Could you check a few things on this model? Use its own coordinates, in mm. Face numbers are marked on the shaded views. A direction names the side the tool comes from. Give positions to 0.01 mm unless a question says otherwise; leave off trailing zeros. Loops run counter-clockwise (first coordinate to the right, second up) from the corner with the lowest first, then second, coordinate; pieces in that order, holes last. Notation, with made-up numbers: (58.5, -25) -> (72.5, -25) arc R14 ccw to (72.5, -4) -> close; hole circle Ø3 at (-3.5, 62.5). An arc over 180 degrees is marked (long way). Write each question's results on one line, items separated by ' | '. Start each with the question number.
Q1. If I drill on line 1 along Z through (x, y) = (84.5, 7.5); line 2 along Y through (x, z) = (11, 51); line 3 along X through (y, z) = (27, 42.5), over which ranges is the centre line in solid material (lowest first)?
Q2. If we section it at B-B, the plane y = 6.5: List the corners of the cut face in (x, z) for me, plus the area to 3 significant figures.
Q3. If we section it at C-C, the plane x = 45.5: List the corners of the cut face in (y, z) for me.
Q4. If we section it at A-A, the plane x = 79: List the corners of the cut face in (y, z) for me, plus the area to 3 significant figures.
Q5. Will these pins go through, and if not, where does the flat tip stop? P1, Ø0.9, axis at y = 2, z = 57, coming from the +X side; P2, Ø10, axis at x = 86, y = 20.5, coming from the -Z side; P3, Ø10, axis at x = 82, y = 14.5, coming from the +Z side.
Q6. If we section it at D-D, the plane z = 31.5: List the corners of the cut face in (x, y) for me, plus the area to 3 significant figures.
Q7. We'd pull the mould along Y, two halves only. Please class the marked faces 1, 2 and 3: released by +Y, released by -Y, zero draft, split by the parting line, or undercut.
Q8. Which directions (+Z, -Z, +X, -X, +Y, -Y) give clear straight access to the entire face, cutting with the end or side of a thin tool? Please do the marked faces 4 and 5.
from build123d import *

# Parameters (mm, degrees)
SKETCH1_R               = 5
BOSS_EXTRUDE1_DEPTH     = 50
SKETCH2_R               = 2
CUT_EXTRUDE1_DEPTH      = 51
SKETCH7_W               = 20
SKETCH7_H               = 39.987182744
CUT_EXTRUDE3_DEPTH      = 10
CUT_EXTRUDE3_DEPTH_BACK = 10
BOSS_EXTRUDE2_REACH     = 52
CUT_EXTRUDE4_REACH      = 97.292
SKETCH9_W               = 20
SKETCH9_H               = 10.896319728
CUT_EXTRUDE6_REACH      = 52
SKETCH11_W              = 5
SKETCH11_H              = 3
SKETCH12_W              = 73
SKETCH12_H              = 70
BOSS_EXTRUDE3_DEPTH     = 3
SKETCH13_W              = 6.758772051
SKETCH13_H              = 20
CUT_EXTRUDE7_DEPTH      = 4


with BuildPart() as part:
    # Sketch1 → Boss-Extrude1 (new body)
    with BuildSketch(Plane.XY):
        with Locations((90.291740814, 26.352640412)):
            Circle(SKETCH1_R)
        Polygon((0, 3), (0, 0), (81.758772051, 0), (91.791740814, 17.924366601), (91.791740814, 23.706854983), (88.791740814, 23.706854983), (88.791740814, 18.706854983), (80, 3), align=None)
    extrude(amount=BOSS_EXTRUDE1_DEPTH)

    # Sketch2 → Cut-Extrude1 (cut, through all)
    with BuildSketch(Plane.XY):
        with Locations((90.291740814, 26.352640412)):
            Circle(SKETCH2_R)
    extrude(amount=CUT_EXTRUDE1_DEPTH, mode=Mode.SUBTRACT)

    # Sketch7 → Cut-Extrude3 (cut, two sides)
    with BuildSketch(Plane(origin=(62.254079791, -34.846042362, 0), x_dir=(0, 0, -1), z_dir=(0.872603055, -0.488430045, 0))) as cut_extrude3_sk:
        with Locations((-25, 59.927032101)):
            Rectangle(SKETCH7_W, SKETCH7_H)
    extrude(amount=CUT_EXTRUDE3_DEPTH, mode=Mode.SUBTRACT)
    extrude(cut_extrude3_sk.sketch, amount=-CUT_EXTRUDE3_DEPTH_BACK, mode=Mode.SUBTRACT)

    # Sketch8 → Boss-Extrude2 (add, up to next)
    with BuildSketch(Plane.XY, mode=Mode.PRIVATE) as boss_extrude2_sk1:
        Polygon((66.951015515, 3), (66.951015515, 0), (81.758772051, 0), (79.25400484, 1.667244856), (80, 3), align=None)
    boss_extrude2_tool1 = extrude(boss_extrude2_sk1.sketch, amount=BOSS_EXTRUDE2_REACH, mode=Mode.PRIVATE) - part.part
    add(boss_extrude2_tool1.solids().sort_by_distance((73.552437, 1.463367, 0))[0])

    # Sketch9 → Cut-Extrude4 (cut, up to next)
    with BuildSketch(Plane(origin=(0, 0, 0), x_dir=(0, 0, -1), z_dir=(1, 0, 0)), mode=Mode.PRIVATE) as cut_extrude4_sk1:
        with Locations((-25, 32.01270193)):
            Rectangle(SKETCH9_W, SKETCH9_H)
    cut_extrude4_tool1 = extrude(cut_extrude4_sk1.sketch, amount=CUT_EXTRUDE4_REACH, mode=Mode.PRIVATE) & part.part
    add(cut_extrude4_tool1.solids().sort_by_distance((0, 32.012702, 25))[0], mode=Mode.SUBTRACT)

    # Sketch11 → Cut-Extrude6 (cut, up to next)
    with BuildSketch(Plane.XY.offset(50), mode=Mode.PRIVATE) as cut_extrude6_sk1:
        with Locations((2.5, 1.5)):
            Rectangle(SKETCH11_W, SKETCH11_H)
    cut_extrude6_tool1 = extrude(cut_extrude6_sk1.sketch, amount=-CUT_EXTRUDE6_REACH, mode=Mode.PRIVATE) & part.part
    add(cut_extrude6_tool1.solids().sort_by_distance((2.5, 1.5, 50))[0], mode=Mode.SUBTRACT)

    # Sketch12 → Boss-Extrude3 (add, through all)
    with BuildSketch(Plane(origin=(0, 3, 0), x_dir=(1, 0, 0), z_dir=(0, 1, 0))):
        with Locations((38.5, -25)):
            Rectangle(SKETCH12_W, SKETCH12_H)
    extrude(amount=-BOSS_EXTRUDE3_DEPTH)

    # Sketch13 → Cut-Extrude7 (cut, through all)
    with BuildSketch(Plane(origin=(0, 3, 0), x_dir=(1, 0, 0), z_dir=(0, 1, 0))):
        with Locations((78.379386025, -25)):
            Rectangle(SKETCH13_W, SKETCH13_H)
    extrude(amount=-CUT_EXTRUDE7_DEPTH, mode=Mode.SUBTRACT)


solid = part.part
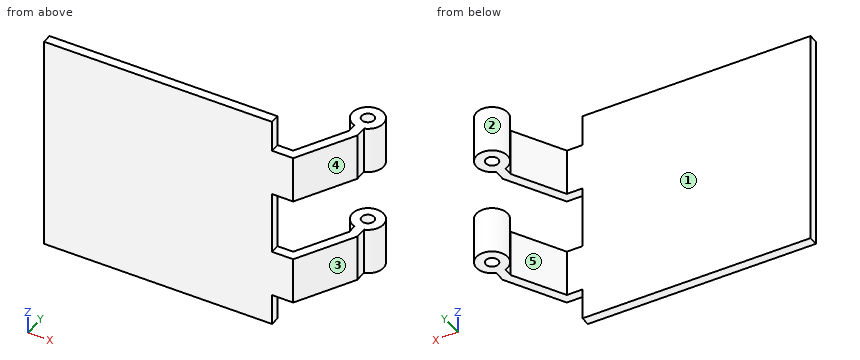
Final values:
1) line 1: z = 0 to 15, 35 to 50 | line 2: y = 0 to 3 | line 3: x = 85.33 to 88.4, 92.18 to 95.25
2) outline: (81.96, 0) -> (85.4, 0) -> (85.4, 15) -> (81.96, 15) -> close; (81.96, 35) -> (85.4, 35) -> (85.4, 50) -> (81.96, 50) -> close | area: 103 mm²
3) outline: (0, -10) -> (3, -10) -> (3, 60) -> (0, 60) -> close
4) outline: (0, 0) -> (3, 0) -> (3, 15) -> (0, 15) -> close; (0, 35) -> (3, 35) -> (3, 50) -> (0, 50) -> close | area: 90.0 mm²
5) P1: stops at x = 75 | P2: stops at z = 0 | P3: stops at z = 50
6) outline: (2, 0) -> (75, 0) -> (75, 3) -> (2, 3) -> close | area: 219 mm²
7) face 1: released by +Y | face 2: undercut | face 3: released by -Y
8) face 4: +Z, -Z, +X, -Y | face 5: +Z, -Z, -X
